from build123d import *

# Parameters (mm, degrees)
F1_DEPTH = 150
F2_W     = 60
F2_H     = 135
F4_R     = 25.991118
F5_DEPTH = 150.001


with BuildPart() as f1:
    # F0 (on Front) → F1 (new body)
    with BuildSketch(Plane.XZ):
        with BuildLine():
            Line((26.036771, 82.488403), (20, 99.074293))
            Line((20, 99.074293), (-20, 99.074293))
            Line((-20, 99.074293), (-26.036771, 82.488403))
            Line((-26.036771, 82.488403), (-39.917332, 76.738886))
            Line((-39.917332, 76.738886), (-71.910606, 91.657595))
            ThreePointArc((-71.910606, 91.657595), (-82.37794, 82.37794), (-91.657595, 71.910606))
            Line((-91.657595, 71.910606), (-76.738886, 39.917332))
            Line((-76.738886, 39.917332), (-82.488403, 26.036771))
            Line((-82.488403, 26.036771), (-115.660184, 13.963229))
            ThreePointArc((-115.660184, 13.963229), (-116.5, 0), (-115.660184, -13.963229))
            Line((-115.660184, -13.963229), (-82.488403, -26.036771))
            Line((-82.488403, -26.036771), (-76.738886, -39.917332))
            Line((-76.738886, -39.917332), (-91.657595, -71.910606))
            ThreePointArc((-91.657595, -71.910606), (-82.37794, -82.37794), (-71.910606, -91.657595))
            Line((-71.910606, -91.657595), (-39.917332, -76.738886))
            Line((-39.917332, -76.738886), (-26.036771, -82.488403))
            Line((-26.036771, -82.488403), (-13.963229, -115.660184))
            ThreePointArc((-13.963229, -115.660184), (0, -116.5), (13.963229, -115.660184))
            Line((13.963229, -115.660184), (26.036771, -82.488403))
            Line((26.036771, -82.488403), (39.917332, -76.738886))
            Line((39.917332, -76.738886), (71.910606, -91.657595))
            ThreePointArc((71.910606, -91.657595), (82.37794, -82.37794), (91.657595, -71.910606))
            Line((91.657595, -71.910606), (76.738886, -39.917332))
            Line((76.738886, -39.917332), (82.488403, -26.036771))
            Line((82.488403, -26.036771), (115.660184, -13.963229))
            ThreePointArc((115.660184, -13.963229), (116.5, 0), (115.660184, 13.963229))
            Line((115.660184, 13.963229), (82.488403, 26.036771))
            Line((82.488403, 26.036771), (76.738886, 39.917332))
            Line((76.738886, 39.917332), (91.657595, 71.910606))
            ThreePointArc((91.657595, 71.910606), (82.37794, 82.37794), (71.910606, 91.657595))
            Line((71.910606, 91.657595), (39.917332, 76.738886))
            Line((39.917332, 76.738886), (26.036771, 82.488403))
        make_face()
        with BuildLine():
            Line((20, 99.074293), (13.963229, 115.660184))
            ThreePointArc((13.963229, 115.660184), (0, 116.5), (-13.963229, 115.660184))
            Line((-13.963229, 115.660184), (-20, 99.074293))
            Line((-20, 99.074293), (20, 99.074293))
        make_face()
    extrude(amount=F1_DEPTH)

    # F2 (on Top) → F3 (revolve, cut)
    with BuildSketch(Plane.XY):
        with Locations((-115.815, -75)):
            Rectangle(F2_W, F2_H)
    revolve(axis=Axis((0, -79.557486, 0), (0, -1, 0)), mode=Mode.SUBTRACT)

    # F4 (on face) → F5 (cut, through all)
    with BuildSketch(Plane.XZ.offset(150)):
        Circle(F4_R)
    extrude(amount=-F5_DEPTH, mode=Mode.SUBTRACT)


solid = f1.part
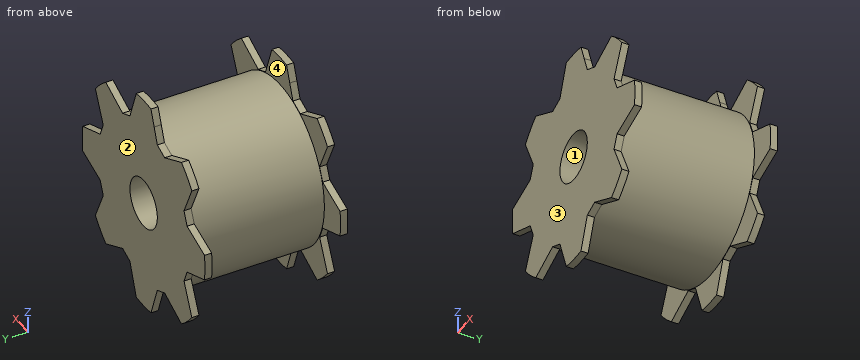
Geometry check sheet. Reference: the model listing, model coordinates, mm. Face numbers are marked on the shaded views. Give positions to 0.01 mm unless a question says otherwise; leave off trailing zeros. Loops run counter-clockwise (first coordinate to the right, second up) from the corner with the lowest first, then second, coordinate; pieces in that order, holes last. Notation, with made-up numbers: M -25.5,58 L 12.5,58 A15 cw 12.5,82 Z; hole C 26,29.25 d6. An arc over 180 degrees is marked long. Write each question's results on one line, items separated by ' | '.
1) Section check C-C, the plane z = -47.5. Record the boundary of the cut face in (x, y).
Answers follow:
outline: M -80.27,-150 L 80.27,-150 L 80.27,-142.5 L 71.47,-142.5 L 71.47,-7.5 L 80.27,-7.5 L 80.27,0 L -80.27,0 L -80.27,-7.5 L -71.47,-7.5 L -71.47,-142.5 L -80.27,-142.5 Z
2) Gauge pin test, flat ends, axial feed: pin 1 (12 mm diameter, centred on x = -12, y = -60.5, fed in from -Z) (3 decimals); pin 2 (3 mm diameter, centred on y = -43, z = -6.5, fed in from +X); pin 3 (12 mm diameter, centred on y = -73.5, z = 33.5, fed in from +X). Record the tip position at first contact, or that the pin passes through.
Answers follow:
pin 1: z = -85.605 | pin 2: x = 85.67 | pin 3: x = 81.29
3) Section check B-B, the plane z = 0. Record the boundary of the cut face in (x, y) (3 decimals).
Answers follow:
outline: M -116.5,-150 L -25.991,-150 L -25.991,0 L -116.5,0 L -116.5,-7.5 L -85.815,-7.5 L -85.815,-142.5 L -116.5,-142.5 Z; M 25.991,-150 L 116.5,-150 L 116.5,-142.5 L 85.815,-142.5 L 85.815,-7.5 L 116.5,-7.5 L 116.5,0 L 25.991,0 Z
4) Release check for a two-part mould opening along Y. For the marked faces 1, 2, 3 and 4 record: +Y half, -Y half, draft (parallel to the pull), parting line (faces both ways), or undercut.
Answers follow:
face 1: draft | face 2: +Y half | face 3: -Y half | face 4: undercut
5) Section check A-A, the plane x = 0. Record the boundary of the cut face in (y, z) (3 decimals).
Answers follow:
outline: M -150,-116.5 L -142.5,-116.5 L -142.5,-85.815 L -7.5,-85.815 L -7.5,-116.5 L 0,-116.5 L 0,-25.991 L -150,-25.991 Z; M -150,25.991 L 0,25.991 L 0,116.5 L -7.5,116.5 L -7.5,85.815 L -142.5,85.815 L -142.5,116.5 L -150,116.5 Z
6) Thickness scan on line 1 (Y direction, x = 20.5, z = -88); line 2 (Z direction, x = 0, y = -80) (3 decimals); line 3 (Z direction, x = -12.5, y = -60). Record the ranges inside material, lowest first.
Answers follow:
line 1: -150 to -142.5, -7.5 to 0 | line 2: -85.815 to -25.991, 25.991 to 85.815 | line 3: -84.9 to -22.79, 22.79 to 84.9
7) Section check D-D, the plane y = -83. Record the boundary of the cut face in (x, z) (3 decimals).
Answers follow:
outline: C 0,0 d171.63; hole C 0,0 d51.982
